```python
from build123d import *

# Parameters (mm, degrees)
F0_R     = 54.9873504391
F0_R_2   = 30.6504677255
F1_DEPTH = 25
F2_DEPTH = 50
F3_SIZE  = 5
F4_DEPTH = 25


with BuildPart() as f1:
    # F0 (on Top) → F1 (new body)
    with BuildSketch(Plane.XY):
        Circle(F0_R)
        Circle(F0_R_2, mode=Mode.SUBTRACT)
    extrude(amount=F1_DEPTH)

    # F2 (add): a face of the model
    f2_faces = [f1.faces().sort_by_distance(p)[0] for p in [
        (-53.4320733041, 0, 25),
    ]]
    extrude(f2_faces, amount=F2_DEPTH)

    # F3
    f3_edges = [f1.edges().sort_by_distance(p)[0] for p in [
        (-54.98735, 0, 75),
    ]]
    chamfer(f3_edges, length=F3_SIZE)

    # F4 (add): a face of the model
    f4_faces = [f1.faces().sort_by_distance(p)[0] for p in [
        (-48.5734946603, 0, 75),
    ]]
    extrude(f4_faces, amount=F4_DEPTH)


solid = f1.part
```
The listing builds one solid part. Answer for the finished solid, in the listing's coordinates (mm). A direction names the side the tool comes from. Round coordinates to 2 decimals unless told otherwise and drop trailing zeros. Loops run counter-clockwise (first coordinate to the right, second up) from the corner with the lowest first, then second, coordinate; pieces in that order, holes last. Notation, with made-up numbers: (89.25, 85.25) -> (145.25, 85.25) arc R19 cw to (145.25, 114.25) -> close; hole circle Ø7 at (19, 40). An arc over 180 degrees is marked (long way). Use one line per item in the form item = value.
1. Flat-ended cylindrical pins translate along their axes: pin 1 Ø1.5 at (x, z) = (6, 11) entering from +Y; pin 2 Ø10 at (x, y) = (16, -33) entering from -Z; pin 3 Ø3 at (x, z) = (-21, 24.5) entering from -Y; pin 4 Ø6 at (y, z) = (-28, 48.5) entering from -X. Find the tip coordinate at first contact, or state that the pin passes through.
Answer key:
pin_1 = 54.74
pin_2 = 0
pin_3 = -51.41
pin_4 = -48.98
2. For a pull along Y with two mould halves and no side action, classify faces 1 (the flat face through (22, 23, 100)), 2 (the conical face through (-6.54, 49.8, 74.76)), 3 (the cylindrical face through (16.478, 25.845, 49.3)) as released by +Y, released by -Y, zero draft, split by the parting line, or undercut.
Answer key:
face_1 = zero draft
face_2 = split by the parting line
face_3 = undercut
3. Find the intervals of material crossed by probe 1 along X at (y, z) = (1, 8); probe 2 along Y at (x, z) = (0, 58.5); probe 3 along Y at (x, z) = (0, 79), in increasing order. Write a range as [from, to].
Answer key:
probe_1 = [-54.98, -30.63], [30.63, 54.98]
probe_2 = [-54.99, -30.65], [30.65, 54.99]
probe_3 = [-49.99, -30.65], [30.65, 49.99]
4. The part is cut by section A-A on y = 0. Determine the outline of the cut face in (x, z).
Answer key:
outline = (-54.99, 0) -> (-30.65, 0) -> (-30.65, 100) -> (-49.99, 100) -> (-49.99, 75) -> (-54.99, 70) -> close; (30.65, 0) -> (54.99, 0) -> (54.99, 70) -> (49.99, 75) -> (49.99, 100) -> (30.65, 100) -> close
5. A tool of negligible diameter and unlimited length cuts with its end or side. For faces 4 (the cylindrical face through (26.87, 42.15, 87.32)), 5 (the cylindrical face through (29.561, 46.366, 34.51)), from which of +Z, -Z, +X, -X, +Y, -Y can it reach the whole face along a straight path? Write none if from no direction.
Answer key:
face_4 = +Z
face_5 = +Z, -Z
6. The part is cut by section D-D on z = 15. Determine the outline of the cut face in (x, y), and give its area (3 significant figures).
Answer key:
outline = circle Ø109.97 at (0, 0); hole circle Ø61.3 at (0, 0)
area = 6,550 mm²
7. The part is cut by section C-C on z = 84. Determine the outline of the cut face in (x, y), and give its area (3 significant figures).
Answer key:
outline = circle Ø99.97 at (0, 0); hole circle Ø61.3 at (0, 0)
area = 4,900 mm²
